from build123d import *

# Parameters (mm, degrees)
F1_DEPTH = 25.4
F0_W     = 25.4
F0_H     = 25.4
F2_DEPTH = 76.2
F3_DEPTH = 50.8


with BuildPart() as f1:
    # F0 (on Top) → F1 (new body)
    with BuildSketch(Plane.XY):
        Polygon((0, 25.4), (0, 0), (25.4, 0), (25.4, 25.4), (50.8, 25.4), (50.8, 50.8), (-25.4, 50.8), (-25.4, 25.4), align=None)
    extrude(amount=F1_DEPTH)

    # F0 (on Top) → F2 (join)
    with BuildSketch(Plane.XY):
        with Locations((-12.7, 12.7)):
            Rectangle(F0_W, F0_H)
    extrude(amount=F2_DEPTH)

    # F0 (on Top) → F3 (join)
    with BuildSketch(Plane.XY):
        with Locations((-12.7, -12.7)):
            Rectangle(F0_W, F0_H)
    extrude(amount=F3_DEPTH)


solid = f1.part
Source: CAD feature listing. Evaluate the final solid. Frame: model axes, mm. A direction names the side the tool comes from. Coordinates: 2 decimals unless noted, no trailing zeros. Order: outer loops, then holes, each group sorted by start corner. A loop starts at its lowest first (then second) coordinate and runs counter-clockwise, first axis right, second up. Notation, with made-up numbers: M 66.5,58.25 L 115.5,58.25 A18 cw 115.5,73.25 Z; hole C -6,-29.5 d4. An arc over 180 degrees is marked long. Write each question's results on one line, items separated by ' | '. Start each with the question number.
Item 1: Line query: probe 1 along X at (y, z) = (-2, 46.5); probe 2 along Z at (x, y) = (-7, 43). Output: solid intervals per line, ascending.
Item 2: Cut plane A-A (z = 18.5). Return loops of the section in (x, y).
Item 3: Set-up query: faces 1 (the face through (-25.4, 4, 29)), 2 (the face through (-13, 25.4, 50)), 3 (the face through (-13, -13, 50.8)), 4 (the face through (25.4, 13, 13)). Return all of +Z, -Z, +X, -X, +Y, -Y with unobstructed straight access to the full face (end or side cutting, diameter ignored); none if empty.
Item 4: First-contact query: pin 1 Ø1.5 at (x, z) = (-2, 54) entering from +Y; pin 2 Ø12.5 at (x, y) = (-7.5, -6.5) entering from +Z; pin 3 Ø1 at (x, z) = (27, 12) entering from -Y. Flat tips, straight axial feed; report the tip coordinate or a pass-through.
Item 5: Cut plane C-C (y = -15.5). Return loops of the section in (x, z).
Item 6: Cut plane B-B (x = -18). Return loops of the section in (y, z).
Item 7: Cut plane D-D (y = 22). Return loops of the section in (x, z), and give its area (3 significant figures).
Checked values:
1) probe 1: x = -25.4 to 0 | probe 2: z = 0 to 25.4
2) outline: M -25.4,-25.4 L 0,-25.4 L 0,0 L 25.4,0 L 25.4,25.4 L 50.8,25.4 L 50.8,50.8 L -25.4,50.8 Z
3) face 1: +Z, -Z, -X, +Y, -Y | face 2: +Z, +X, -X, +Y | face 3: +Z, +X, -X, -Y | face 4: +Z, -Z, +X, -Y
4) pin 1: stops at y = 25.4 | pin 2: stops at z = 50.8 | pin 3: stops at y = 25.4
5) outline: M -25.4,0 L 0,0 L 0,50.8 L -25.4,50.8 Z
6) outline: M -25.4,0 L 50.8,0 L 50.8,25.4 L 25.4,25.4 L 25.4,76.2 L 0,76.2 L 0,50.8 L -25.4,50.8 Z
7) outline: M -25.4,0 L 25.4,0 L 25.4,25.4 L 0,25.4 L 0,76.2 L -25.4,76.2 Z | area: 2,580 mm2
